```python
from build123d import *

# Parameters (mm, degrees)
SKETCH_1_W          = 6
SKETCH_1_H          = 70
EXTRUDE_1_DEPTH     = 6
SKETCH_4_R          = 1.25
CUT_EXTRUDE_3_DEPTH = 8
SKETCH_6_R          = 1.2
CUT_EXTRUDE_5_DEPTH = 10
SKETCH_7_W          = 6
SKETCH_7_H          = 6
CUT_EXTRUDE_6_DEPTH = 20


with BuildPart() as part:
    # 草图1 → 凸台-拉伸1 (new body)
    with BuildSketch(Plane.XY):
        with Locations((3, 35)):
            Rectangle(SKETCH_1_W, SKETCH_1_H)
    extrude(amount=EXTRUDE_1_DEPTH)

    # 草图4 → 切除-拉伸3 (cut)
    with BuildSketch(Plane.ZY):
        with Locations((3, 65)):
            Circle(SKETCH_4_R)
        with Locations((3, 45)):
            Circle(SKETCH_4_R)
        with Locations((3, 25)):
            Circle(SKETCH_4_R)
        with Locations((3, 5)):
            Circle(SKETCH_4_R)
    extrude(amount=-CUT_EXTRUDE_3_DEPTH, mode=Mode.SUBTRACT)

    # 草图6 → 切除-拉伸5 (cut)
    with BuildSketch(Plane.XY.offset(6)):
        with Locations((3, 15)):
            Circle(SKETCH_6_R)
        with Locations((3, 35)):
            Circle(SKETCH_6_R)
        with Locations((3, 55)):
            Circle(SKETCH_6_R)
    extrude(amount=-CUT_EXTRUDE_5_DEPTH, mode=Mode.SUBTRACT)

    # 草图7 → 切除-拉伸6 (cut)
    with BuildSketch(Plane(origin=(0, 70, 0), x_dir=(1, 0, 0), z_dir=(0, 1, 0))):
        with Locations((3, -3)):
            Rectangle(SKETCH_7_W, SKETCH_7_H)
    extrude(amount=-CUT_EXTRUDE_6_DEPTH, mode=Mode.SUBTRACT)


solid = part.part
```
Geometry: final body of the model. Coordinates: model frame, mm. Coordinates: 2 decimals unless noted, no trailing zeros. Loops run counter-clockwise (first coordinate to the right, second up) from the corner with the lowest first, then second, coordinate; pieces in that order, holes last. Notation, with made-up numbers: (57, 88) -> (92, 88) arc R11 cw to (92, 98) -> close; hole circle Ø1 at (-32.5, -39). An arc over 180 degrees is marked (long way). Use a Markdown table: item, result. Add a question column.
(1) Section query A-A, the plane z = 3. Return loops of the section in (x, y), plus the area to 3 significant figures.
(2) Section query B-B, the plane y = 35. Return loops of the section in (x, z).
(3) Mould query, pull axis Z, two halves, no side actions, for faces 1 (the flat face through (3, 25, 0)), 2 (the cylindrical face through (2.958, 3.891, 3.577)), 3 (the cylindrical face through (2.96, 25.38, 4.19)), 4 (the cylindrical face through (2.74, 13.83, 3.04)). Classes: pulls with the +Z half, pulls with the -Z half, needs draft (parallel to the pull), parting line crosses it, or undercut.
(4) Section query D-D, the plane x = 2.5. Return loops of the section in (y, z).
(5) Pin query (flat end, axial travel): pin 1 Ø2 at (y, z) = (5, 3) entering from +X. Return the tip coordinate at first contact, or that it passes through.
(6) Section query C-C, the plane x = 0.6. Return loops of the section in (y, z).
(7) Line query: line 1 along Y through (x, z) = (3.4, 1.3); line 2 along Y through (x, z) = (2.15, 2.55); line 3 along Y through (x, z) = (3.4, 2.1). Output: solid intervals per line, ascending.
Answer:
| question | item | result |
|---|---|---|
| 1 | outline | (0, 0) -> (6, 0) -> (6, 3.75) -> (0, 3.75) -> close; (0, 6.25) -> (6, 6.25) -> (6, 23.75) -> (0, 23.75) -> close; (0, 26.25) -> (6, 26.25) -> (6, 43.75) -> (0, 43.75) -> close; (0, 46.25) -> (6, 46.25) -> (6, 50) -> (0, 50) -> close; hole circle Ø2.4 at (3, 15); hole circle Ø2.4 at (3, 35) |
| 1 | area | 246 mm^2 |
| 2 | outline | (0, 0) -> (1.8, 0) -> (1.8, 6) -> (0, 6) -> close; (4.2, 0) -> (6, 0) -> (6, 6) -> (4.2, 6) -> close |
| 3 | face 1 | pulls with the -Z half |
| 3 | face 2 | undercut |
| 3 | face 3 | undercut |
| 3 | face 4 | needs draft |
| 4 | outline | (0, 0) -> (13.91, 0) -> (13.91, 6) -> (0, 6) -> close; (16.09, 0) -> (33.91, 0) -> (33.91, 6) -> (16.09, 6) -> close; (36.09, 0) -> (50, 0) -> (50, 6) -> (36.09, 6) -> close; hole circle Ø2.5 at (5, 3); hole circle Ø2.5 at (25, 3); hole circle Ø2.5 at (45, 3) |
| 5 | pin 1 | passes through |
| 6 | outline | (0, 0) -> (50, 0) -> (50, 6) -> (0, 6) -> close; hole circle Ø2.5 at (5, 3); hole circle Ø2.5 at (25, 3); hole circle Ø2.5 at (45, 3) |
| 7 | line 1 | y = 0 to 13.87, 16.13 to 33.87, 36.13 to 50 |
| 7 | line 2 | y = 0 to 3.83, 6.17 to 14.15, 15.85 to 23.83, 26.17 to 34.15, 35.85 to 43.83, 46.17 to 50 |
| 7 | line 3 | y = 0 to 4.13, 5.87 to 13.87, 16.13 to 24.13, 25.87 to 33.87, 36.13 to 44.13, 45.87 to 50 |
